```python
from build123d import *

# Parameters (mm, degrees)
F0_W         = 27
F0_H         = 22
F1_DEPTH     = 20
F2_W         = 21
F2_H         = 21
F3_DEPTH     = 6
F5_DEPTH     = 2
F7_DEPTH     = 20
F8_DEPTH     = 6
F9_W         = 27
F9_H         = 22
F10_DEPTH    = 3
F11_T1_DEPTH = 52.7168298797
F12_R        = 8.5
F13_DEPTH    = 20
F14_DEPTH    = 1


# Not quite as in the source:
# - a fillet or chamfer that OpenCascade refuses, or shapes differently, is made with other operations: its cross-section is extruded or revolved along the edge and cut away or added


with BuildPart() as f1:
    # F0 (on Top) → F1 (new body)
    with BuildSketch(Plane.XY):
        Rectangle(F0_W, F0_H)
    extrude(amount=F1_DEPTH)

    # F2 (on face) → F3 (cut)
    with BuildSketch(Plane(origin=(0, 0, 0), x_dir=(1, 0, 0), z_dir=(0, 0, -1))):
        with Locations((0, 0.5)):
            Rectangle(F2_W, F2_H)
    extrude(amount=-F3_DEPTH, mode=Mode.SUBTRACT)

    # F4 (on face) → F5 (cut)
    with BuildSketch(Plane(origin=(0, 0, 6), x_dir=(1, 0, 0), z_dir=(0, 0, -1))):
        Polygon((0, 11), (-7, 11), (-7, -11), (7, -11), (7, 11), align=None)
    extrude(amount=-F5_DEPTH, mode=Mode.SUBTRACT)

    # F6 (on face) → F7 (cut)
    with BuildSketch(Plane.XY.offset(20)):
        Polygon((0, -3), (3, -3), (3, 3), (-3, 3), (-3, -3), align=None)
    extrude(amount=-F7_DEPTH, mode=Mode.SUBTRACT)

    # F8 (cut): a face of the model
    f8_faces = [f1.faces().sort_by_distance(p)[0] for p in [
        (0, 10.5, 6),
    ]]
    extrude(f8_faces, amount=-F8_DEPTH, mode=Mode.SUBTRACT)

    # F9 (on face) → F10 (join)
    with BuildSketch(Plane(origin=(0, 0, 0), x_dir=(1, 0, 0), z_dir=(0, 0, -1))):
        Rectangle(F9_W, F9_H)
    extrude(amount=F10_DEPTH)

    # F11: chamfer of 5 on 1 edges, made by hand

    # F11_s2 → F11_t1 (cut)
    with BuildSketch(Plane.YZ.offset(-26.3584149398)):
        Polygon((11, 2), (6, -3), (11, -3), align=None)
    extrude(amount=F11_T1_DEPTH, mode=Mode.SUBTRACT)

    # F12 (on face) → F13 (cut)
    with BuildSketch(Plane.XY.offset(20)):
        Circle(F12_R)
    extrude(amount=-F13_DEPTH, mode=Mode.SUBTRACT)

    # F14 (cut): faces of the model
    f14_faces = [f1.faces().sort_by_distance(p)[0] for p in [
        (-8.9267642555, -0.5771749807, 6),
        (8.9267642555, -0.5771749807, 6),
        (0, -9.0505273171, 8),
        (0, 9.0505273171, 8),
    ]]
    extrude(f14_faces, amount=-F14_DEPTH, mode=Mode.SUBTRACT)


solid = f1.part
```
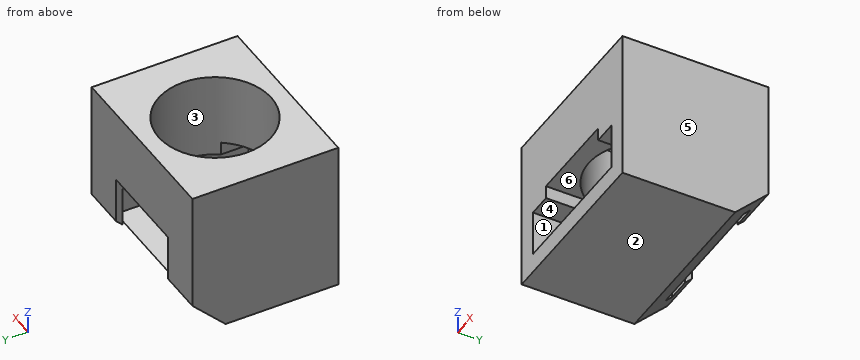
Can you work these out from the model? Positions are in its coordinate system, mm. Face numbers are marked on the shaded views. A direction names the side the tool comes from. Give positions to 0.01 mm unless a question says otherwise; leave off trailing zeros. Loops run counter-clockwise (first coordinate to the right, second up) from the corner with the lowest first, then second, coordinate; pieces in that order, holes last. Notation, with made-up numbers: M -27.75,27.5 L 19.25,27.5 A8 cw 19.25,36.5 Z; hole C 14,75.25 d8. An arc over 180 degrees is marked long. Answer in a Markdown table with one row per item.
1. If I drill on line 1 along Y through (x, z) = (0, 13.5); line 2 along X through (y, z) = (-7, 3.5); line 3 along X through (y, z) = (0, 12.5), over which ranges is the centre line in solid material (lowest first)?
Taken from the geometry:
| item | result |
|---|---|
| line 1 | y = -11 to -8.5, 8.5 to 11 |
| line 2 | x = -13.5 to -10.5, 10.5 to 13.5 |
| line 3 | x = -13.5 to -8.5, 8.5 to 13.5 |
2. Suppose I cut it at C-C on z = 13.5. Write out the boundary of the cut face in (x, y).
Taken from the geometry:
| item | result |
|---|---|
| outline | M -13.5,-11 L 13.5,-11 L 13.5,11 L -13.5,11 Z; hole C 0,0 d17 |
3. Suppose I cut it at A-A on x = 0. Write out the boundary of the cut face in (y, z), plus the area to 4 significant figures.
Taken from the geometry:
| item | result |
|---|---|
| outline | M -11,-3 L 6,-3 L 9,0 L -11,0 Z; M -11,9 L -8.5,9 L -8.5,20 L -11,20 Z; M 8.5,9 L 11,9 L 11,20 L 8.5,20 Z |
| area | 110.5 mm² |
4. Suppose I cut it at D-D on x = -6.5. Write out the boundary of the cut face in (y, z).
Taken from the geometry:
| item | result |
|---|---|
| outline | M -11,-3 L 6,-3 L 9,0 L -11,0 Z; M -11,9 L -5.48,9 L -5.48,20 L -11,20 Z; M 5.48,9 L 11,9 L 11,20 L 5.48,20 Z |
5. For pin 1 Ø10 at (x, z) = (-3, 8) entering from +Y; pin 2 Ø1.8 at (x, z) = (8.5, 5.5) entering from -Y, each with a flat end and sliding along its axis, tell me the tip position at first contact or that it passes through.
Taken from the geometry:
| item | result |
|---|---|
| pin 1 | stops at y = 11 |
| pin 2 | stops at y = 10 |
6. Thinking about a two-plate mould opening in Z: for the marked faces 1, 2 and 3, which applies, released by +Z, released by -Z, zero draft, split by the parting line, or undercut?
Taken from the geometry:
| item | result |
|---|---|
| face 1 | undercut |
| face 2 | released by -Z |
| face 3 | zero draft |
7. Suppose I cut it at B-B on y = 0. Write out the boundary of the cut face in (x, z), plus the area to 3 significant figures.
Taken from the geometry:
| item | result |
|---|---|
| outline | M -13.5,-3 L 13.5,-3 L 13.5,20 L 8.5,20 L 8.5,7 L 10.5,7 L 10.5,0 L -10.5,0 L -10.5,7 L -8.5,7 L -8.5,20 L -13.5,20 Z |
| area | 253 mm² |
8. Which directions (+Z, -Z, +X, -X, +Y, -Y) give clear straight access to the entire face, cutting with the end or side of a thin tool? Please do the marked faces 4, 5 and 6.
Taken from the geometry:
| item | result |
|---|---|
| face 4 | -Y |
| face 5 | +Z, -Z, +X, +Y, -Y |
| face 6 | +Y, -Y |
